Print and shaded views of the part. All mm, measured from the part's lowest x, y and z. A direction names the side the tool comes from. Coordinates: 2 decimals unless noted, no trailing zeros. Order: outer loops, then holes, each group sorted by start corner. A loop starts at its lowest first (then second) coordinate and runs counter-clockwise, first axis right, second up.
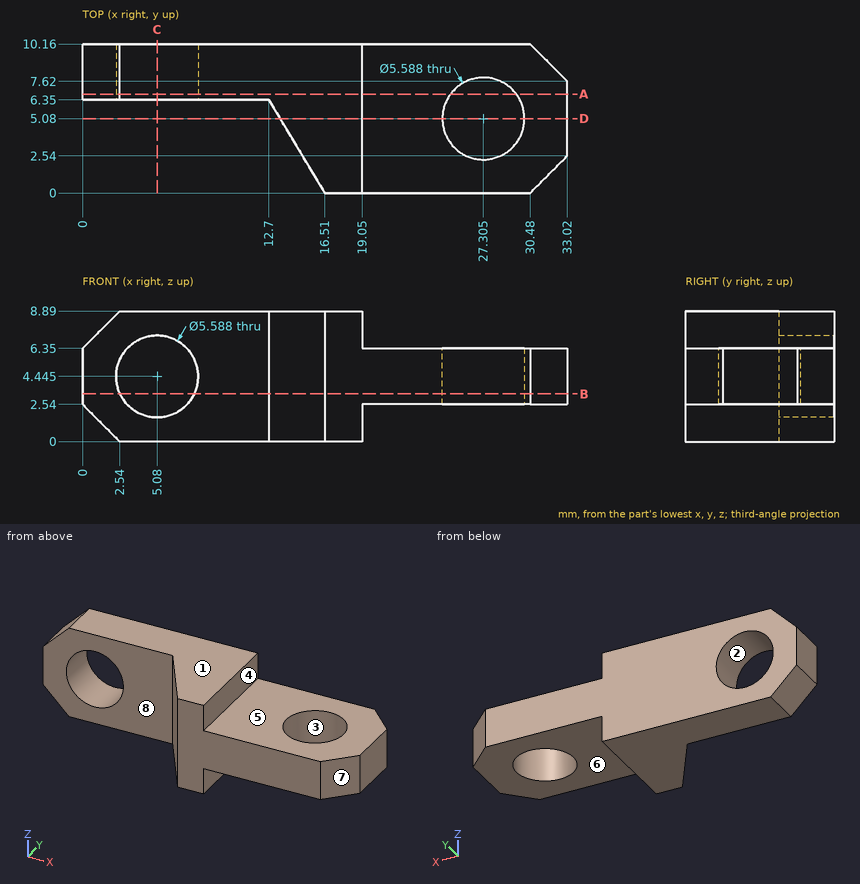
Q1. Probe line 1 (Z direction, x = 5.08, y = 7.85); line 2 (Y direction, x = 11.5, z = 6.75); line 3 (X direction, y = 7.75, z = 8). List the from-to ranges inside material, lowest first.
Established:
line 1: z = 0 to 1.65, 7.24 to 8.89
line 2: y = 6.35 to 10.16
line 3: x = 1.65 to 19.05
Q2. Mould opens along X. For the marked faces 1, 2, 3 and 4 say: pulls with the +X half, pulls with the -X half, needs draft (parallel to the pull), parting line crosses it, or undercut.
Established:
face 1: needs draft
face 2: undercut
face 3: undercut
face 4: pulls with the +X half
Q3. Which spindle directions (+Z, -Z, +X, -X, +Y, -Y) get a long thin tool onto all of the face, cutting with end or side? Do the marked faces 5, 6, 7 and 8. Say none if no direction does.
Established:
face 5: +Z, +X, +Y, -Y
face 6: -Z, +X, +Y, -Y
face 7: +Z, -Z, +X, -Y
face 8: +Z, -Z, -X, -Y
Q4. Cut at C-C, the plane x = 5.08. List the corners of the cut face in (y, z), plus the area to 3 significant figures.
Established:
outline: (6.35, 0) - (10.16, 0) - (10.16, 1.65) - (6.35, 1.65) - close; (6.35, 7.24) - (10.16, 7.24) - (10.16, 8.89) - (6.35, 8.89) - close
area: 12.6 mm2
Q5. Cut at A-A, the plane y = 6.75. List the corners of the cut face in (x, z) (3 decimals), plus the area to 3 significant figures.
Established:
outline: (0, 2.54) - (2.54, 0) - (19.05, 0) - (19.05, 2.54) - (25.065, 2.54) - (25.065, 6.35) - (19.05, 6.35) - (19.05, 8.89) - (2.54, 8.89) - (0, 6.35) - close; (29.545, 2.54) - (33.02, 2.54) - (33.02, 6.35) - (29.545, 6.35) - close; hole circle Ø5.588 at (5.08, 4.445)
area: 175 mm2
Q6. Cut at B-B, the plane z = 3.25. List the corners of the cut face in (x, y) (3 decimals), plus the area to 3 significant figures.
Established:
outline: (0, 6.35) - (2.554, 6.35) - (2.554, 10.16) - (0, 10.16) - close; (7.606, 6.35) - (12.7, 6.35) - (16.51, 0) - (30.48, 0) - (33.02, 2.54) - (33.02, 7.62) - (30.48, 10.16) - (7.606, 10.16) - close; hole circle Ø5.588 at (27.305, 5.08)
area: 193 mm2
Q7. Drop flat-ended pins along their axis: P1, Ø1.3, axis at y = 4, z = 1.5, coming from the +X side; P2, Ø5, axis at x = 27.305, y = 5.08, coming from the -Z side; P3, Ø5, axis at x = 23, y = 4.5, coming from the -Z side; P4, Ø2.5, axis at x = 5, z = 2.5, coming from the -Y side. Give the stop position or say it passes through.
Established:
P1: stops at x = 19.05
P2: passes through
P3: stops at z = 2.54
P4: stops at y = 6.35
Q8. Cut at D-D, the plane y = 5.08. List the corners of the cut face in (x, z).
Established:
outline: (13.46, 0) - (19.05, 0) - (19.05, 2.54) - (24.51, 2.54) - (24.51, 6.35) - (19.05, 6.35) - (19.05, 8.89) - (13.46, 8.89) - close; (30.1, 2.54) - (33.02, 2.54) - (33.02, 6.35) - (30.1, 6.35) - close
